Geometry check sheet. Reference: drawing and pictorial views, mm from the part's lowest x, y, z. Give positions to 0.01 mm unless a question says otherwise; leave off trailing zeros. Loops run counter-clockwise (first coordinate to the right, second up) from the corner with the lowest first, then second, coordinate; pieces in that order, holes last. Notation, with made-up numbers: (66, 42.5) -> (106, 42.5) arc R21 cw to (106, 74.5) -> close; hole circle Ø2 at (75.25, 26). An arc over 180 degrees is marked (long way). One line per item, written item: value. Start each with the question number.
(1) Gauge pin test, flat ends, axial feed: pin 1 Ø20 at (x, y) = (33, 240) entering from +Z; pin 2 Ø3.5 at (y, z) = (107.5, 15) entering from +X; pin 3 Ø5 at (y, z) = (95.5, 12.5) entering from -X; pin 4 Ø4 at (x, y) = (22.5, 35) entering from -Z. Record the tip position at first contact, or that the pin passes through.
(2) Sectioned sample at A-A, the plane y = 78.5. Record the cut outline in (x, z), then the cut area to 3 significant figures.
(3) Draft check along Y on the marked faces 1, 2 and 3. Enter one of: pulls with the +Y half, pulls with the -Y half, needs draft (parallel to the pull), parting line crosses it, or undercut.
(4) Sectioned sample at B-B, the plane x = 32.5. Record the cut outline in (y, z).
(5) Scan lines: line 1 along Y through (x, z) = (22.5, 7); line 2 along Y through (x, z) = (21, 7.75); line 3 along Z through (x, y) = (28, 114). Record each from-to range of solid material in increasing order. Write a range as from..to.
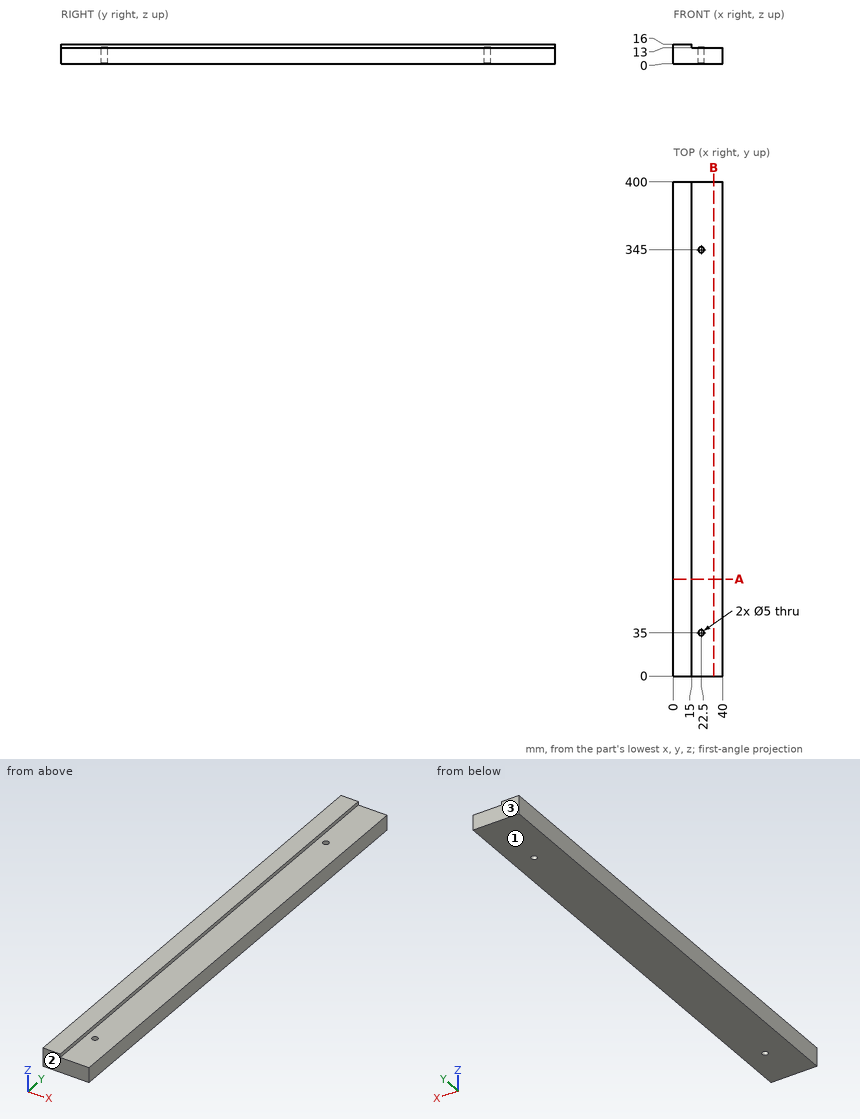
Calculated:
1. pin 1: stops at z = 13
1. pin 2: stops at x = 15
1. pin 3: stops at x = 0
1. pin 4: passes through
2. outline: (0, 0) -> (40, 0) -> (40, 13) -> (15, 13) -> (15, 16) -> (0, 16) -> close
2. area: 565 mm2
3. face 1: needs draft
3. face 2: pulls with the -Y half
3. face 3: pulls with the +Y half
4. outline: (0, 0) -> (400, 0) -> (400, 13) -> (0, 13) -> close
5. line 1: y = 0..32.5, 37.5..342.5, 347.5..400
5. line 2: y = 0..33, 37..343, 347..400
5. line 3: z = 0..13
